from build123d import *

# Parameters (mm, degrees)
SKETCH2_R               = 8
BOSS_EXTRUDE1_DEPTH     = 26
CUT_EXTRUDE1_DEPTH      = 29.354893758
CUT_EXTRUDE1_DEPTH_BACK = 29.354893758
SKETCH3_R               = 3.5
SKETCH4_R               = 1.5
BOSS_EXTRUDE2_DEPTH     = 15
SKETCH6_R               = 7
BOSS_EXTRUDE3_DEPTH     = 20


with BuildPart() as part:
    # Sketch2 → Boss-Extrude1 (new body)
    with BuildSketch(Plane(origin=(0, 0, 0), x_dir=(1, 0, 0), z_dir=(0, 1, 0))):
        with Locations(Location((0, 0, 0), (0, 0, 90))):
            Circle(SKETCH2_R)
    extrude(amount=BOSS_EXTRUDE1_DEPTH)

    # Sketch3 → Cut-Extrude1 (cut, two sides: drawn at the far end of the back side and taken through both)
    with BuildSketch(Plane(origin=(0, 0, 0), x_dir=(0, 0, -1), z_dir=(1, 0, 0)).offset(-CUT_EXTRUDE1_DEPTH_BACK)):
        with Locations((0, 5.5)):
            Circle(SKETCH3_R)
    extrude(amount=CUT_EXTRUDE1_DEPTH + CUT_EXTRUDE1_DEPTH_BACK, mode=Mode.SUBTRACT)

    # Sketch4 → Boss-Extrude2 (add)
    with BuildSketch(Plane(origin=(0, 0, 0), x_dir=(0, 0, -1), z_dir=(1, 0, 0))):
        with Locations(Location((0, 20.5, 0), (0, 0, 180))):
            Circle(SKETCH4_R)
    extrude(amount=BOSS_EXTRUDE2_DEPTH)

    # Sketch6 → Boss-Extrude3 (add)
    with BuildSketch(Plane(origin=(0, 26, 0), x_dir=(1, 0, 0), z_dir=(0, 1, 0))):
        with Locations(Location((0, 0, 0), (0, 0, 270))):
            Circle(SKETCH6_R)
    extrude(amount=BOSS_EXTRUDE3_DEPTH)


solid = part.part
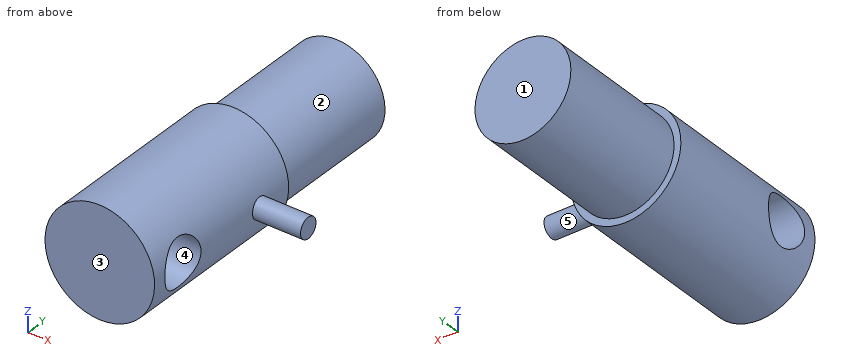
For this review, take the finished solid that the model builds, in its own axes (mm). Face numbers are marked on the shaded views. A direction names the side the tool comes from. Coordinates: 2 decimals unless noted, no trailing zeros. Write each loop counter-clockwise with the first axis right and the second up, starting at its lowest first coordinate (ties: lowest second). Pieces come first, ordered by that corner, then holes. Notation, with made-up numbers: (38, -24) -> (56, -24) arc R9 ccw to (56, -15) -> close; hole circle Ø10 at (74.5, 79). An arc over 180 degrees is marked (long way). Write each question's results on one line, items separated by ' | '. Start each with the question number.
1) Consider section C-C (y = 5.5). Write out the cut boundary in (x, z).
2) For the marked faces 1 and 2, list the 3-axis set-ups (+Z, -Z, +X, -X, +Y, -Y) from which the entire face can be reached by the end or side of a thin tool; tool diameter is ignored.
3) Consider section B-B (z = 0). Write out the cut boundary in (x, y), plus the area to 3 significant figures.
4) Wall thickness on L1, parallel to Y at x = -0.25, z = 0; L2, parallel to Y at x = 2.5, z = 1; L3, parallel to Z at x = -7, y = 6: over which ranges is each line inside the solid? List them lowest first. Write a range as [from, to].
5) The part is to be moulded in two halves that separate along Y. For the marked faces 3, 4 and 5, say which applies: +Y half, -Y half, draft (parallel to the pull), parting line (faces both ways), or undercut.
6) Consider section D-D (z = -5). Write out the cut boundary in (x, y) (3 decimals), plus the area to 3 significant figures.
7) Insertion check: pin 1 (4 mm diameter, centred on x = 11.5, y = 12.5, fed in from +Z); pin 2 (5 mm diameter, centred on x = 11.5, y = 23, fed in from +Z); pin 3 (1.5 mm diameter, centred on x = 1, y = 12.5, fed in from +Z); pin 4 (8 mm diameter, centred on y = 20, z = -1, fed in from -X). Each pin has a flat end and moves straight along its axis. Give the tip position at first contact, or say it passes through.
8) Consider section A-A (x = 0). Write out the cut boundary in (y, z).
Geometry says:
1) outline: (-7.19, -3.5) arc R8 ccw to (7.19, -3.5) -> close; (-7.19, 3.5) -> (7.19, 3.5) arc R8 ccw to start
2) face 1: +Z, -Z, +X, -X, +Y | face 2: +Y
3) outline: (-8, 0) -> (8, 0) -> (8, 2) -> (-8, 2) -> close; (-8, 9) -> (8, 9) -> (8, 19) -> (15, 19) -> (15, 22) -> (8, 22) -> (8, 26) -> (7, 26) -> (7, 46) -> (-7, 46) -> (-7, 26) -> (-8, 26) -> close | area: 605 mm^2
4) L1: [0, 2], [9, 46] | L2: [0, 2.15], [8.85, 46] | L3: [-3.87, -3.46], [3.46, 3.87]
5) face 3: -Y half | face 4: undercut | face 5: parting line
6) outline: (-6.245, 0) -> (6.245, 0) -> (6.245, 26) -> (4.899, 26) -> (4.899, 46) -> (-4.899, 46) -> (-4.899, 26) -> (-6.245, 26) -> close | area: 521 mm^2
7) pin 1: through | pin 2: z = 1.5 | pin 3: z = 8 | pin 4: x = -8
8) outline: (0, -8) -> (26, -8) -> (26, -7) -> (46, -7) -> (46, 7) -> (26, 7) -> (26, 8) -> (0, 8) -> close; hole circle Ø7 at (5.5, 0)
